Work out the finished part from the listing and answer in its coordinate system (mm). A direction names the side the tool comes from. Coordinates: 2 decimals unless noted, no trailing zeros. Order: outer loops, then holes, each group sorted by start corner. A loop starts at its lowest first (then second) coordinate and runs counter-clockwise, first axis right, second up. Notation, with made-up numbers: (-23.75, 61) - (0.25, 61) arc R23 ccw to (0.25, 72) - close; hole circle Ø5 at (74.25, 46). An arc over 180 degrees is marked (long way). Use CSV: the item, a comma, the result in double quotes. Start each with the question number.
from build123d import *

# Parameters (mm, degrees)
CYLINDER028_R          = 4
CYLINDER028_DEPTH      = 2.5
CYLINDER028_ROLL_ANGLE = 90
BOX023_W               = 5
BOX023_H               = 2.5
BOX023_DEPTH           = 2.5
CHAMFER003_SIZE        = 2.49
BOX021_W               = 5
BOX021_H               = 2.5
BOX021_DEPTH           = 2.5
CHAMFER001_SIZE        = 2.49
CYLINDER014_R          = 0.8
CYLINDER014_DEPTH      = 28
CYLINDER015_R          = 0.8
CYLINDER015_DEPTH      = 28
CYLINDER009_R          = 0.8
CYLINDER009_DEPTH      = 28
CYLINDER008_R          = 0.8
CYLINDER008_DEPTH      = 28
BOX012_W               = 73
BOX012_H               = 37
BOX012_DEPTH           = 3
BOX011_W               = 73
BOX011_H               = 3
BOX011_DEPTH           = 8
FILLET004_R            = 7.99
FILLET005_R            = 2


with BuildPart() as cylinder028:
    # Cylinder028 → Cylinder028 (new body)
    with BuildSketch(Plane.XY):
        Circle(CYLINDER028_R)
    extrude(amount=CYLINDER028_DEPTH)


with BuildPart() as cylinder028_1:
    # Cylinder028 roll: moved
    add(cylinder028.part.rotate(Axis((0, 0, 0), (1, 0, 0)), CYLINDER028_ROLL_ANGLE))


with BuildPart() as cylinder028_2:
    # Cylinder028 placement: moved
    add(cylinder028_1.part.moved(Location((63, 84.5, -17))))


with BuildPart() as chamfer003:
    # Box023 → Box023 (new body)
    with BuildSketch(Plane(origin=(70.5, 113, -22.5), x_dir=(1, 0, 0), z_dir=(0, 0, 1))):
        with Locations((2.5, 1.25)):
            Rectangle(BOX023_W, BOX023_H)
    extrude(amount=BOX023_DEPTH)

    # Chamfer003
    chamfer003_edges = [chamfer003.edges().sort_by_distance(p)[0] for p in [
        (73, 115.5, -22.5),
    ]]
    chamfer(chamfer003_edges, length=CHAMFER003_SIZE)


with BuildPart() as chamfer003_1:
    # Chamfer003 placement: moved
    add(chamfer003.part.moved(Location((55, 9, 0))))


with BuildPart() as fusion016:
    # Box021 → Box021 (new body)
    with BuildSketch(Plane(origin=(70.5, 113, -22.5), x_dir=(1, 0, 0), z_dir=(0, 0, 1))):
        with Locations((2.5, 1.25)):
            Rectangle(BOX021_W, BOX021_H)
    extrude(amount=BOX021_DEPTH)

    # Chamfer001
    chamfer001_edges = [fusion016.edges().sort_by_distance(p)[0] for p in [
        (73, 115.5, -22.5),
    ]]
    chamfer(chamfer001_edges, length=CHAMFER001_SIZE)


with BuildPart() as fusion016_1:
    # Chamfer001 placement: moved
    add(fusion016.part.moved(Location((1, 9, 0))))

    # Fusion016: union Chamfer003
    add(chamfer003_1.part)


with BuildPart() as cylinder014:
    # Cylinder014 → Cylinder014 (new body)
    with BuildSketch(Plane(origin=(74, 118, -26), x_dir=(1, 0, 0), z_dir=(0, 0, 1))):
        Circle(CYLINDER014_R)
    extrude(amount=CYLINDER014_DEPTH)


with BuildPart() as fusion011:
    # Cylinder015 → Cylinder015 (new body)
    with BuildSketch(Plane(origin=(74, 94, -26), x_dir=(1, 0, 0), z_dir=(0, 0, 1))):
        Circle(CYLINDER015_R)
    extrude(amount=CYLINDER015_DEPTH)

    # Fusion011: union Cylinder014
    add(cylinder014.part)


with BuildPart() as fusion011_1:
    # Fusion011 placement: moved
    add(fusion011.part.moved(Location((54, 0, 0))))


with BuildPart() as cylinder009:
    # Cylinder009 → Cylinder009 (new body)
    with BuildSketch(Plane(origin=(74, 118, -26), x_dir=(1, 0, 0), z_dir=(0, 0, 1))):
        Circle(CYLINDER009_R)
    extrude(amount=CYLINDER009_DEPTH)


with BuildPart() as fusion012:
    # Cylinder008 → Cylinder008 (new body)
    with BuildSketch(Plane(origin=(74, 94, -26), x_dir=(1, 0, 0), z_dir=(0, 0, 1))):
        Circle(CYLINDER008_R)
    extrude(amount=CYLINDER008_DEPTH)

    # Fusion010: union Cylinder009
    add(cylinder009.part)

    # Fusion012: union Fusion011
    add(fusion011_1.part)


with BuildPart() as box012:
    # Box012 → Box012 (new body)
    with BuildSketch(Plane(origin=(64, 85, -23), x_dir=(1, 0, 0), z_dir=(0, 0, 1))):
        with Locations((36.5, 18.5)):
            Rectangle(BOX012_W, BOX012_H)
    extrude(amount=BOX012_DEPTH)


with BuildPart() as cut026:
    # Box011 → Box011 (new body)
    with BuildSketch(Plane(origin=(64, 82, -23), x_dir=(1, 0, 0), z_dir=(0, 0, 1))):
        with Locations((36.5, 1.5)):
            Rectangle(BOX011_W, BOX011_H)
    extrude(amount=BOX011_DEPTH)

    # Fusion001: union Box012
    add(box012.part)

    # Fillet004
    fillet004_edges = [cut026.edges().sort_by_distance(p)[0] for p in [
        (100.5, 82, -23),
    ]]
    fillet(fillet004_edges, radius=FILLET004_R)

    # Fillet005
    fillet005_edges = [cut026.edges().sort_by_distance(p)[0] for p in [
        (100.5, 85, -20),
    ]]
    fillet(fillet005_edges, radius=FILLET005_R)

    # Cut013: cut Fusion012
    add(fusion012.part, mode=Mode.SUBTRACT)

    # Fusion017: union Fusion016
    add(fusion016_1.part)

    # Cut026: cut Cylinder028
    add(cylinder028_2.part, mode=Mode.SUBTRACT)


solid = cut026.part
1) The part is cut by section A-A on y = 118. Determine the outline of the cut face in (x, z).
2) The part is cut by section C-C on z = -21.5. Determine the outline of the cut face in (x, y).
3) For a pull along Z with two mould halves and no side action, classify faces 1 (the face through (76.5, 123, -21)), 2 (the face through (66.932, 83.545, -17.735)), 3 (the face through (100, 106, -20)) as +Z half, -Z half, draft (parallel to the pull), parting line (faces both ways), or undercut.
4) Flat-ended cylindrical pins translate along their axes: P1, Ø11, axis at x = 91, y = 97.5, coming from the +Z side; P2, Ø1.5, axis at x = 86.5, z = -17, coming from the +Y side; P3, Ø2, axis at x = 105, z = -17, coming from the -Y side; P4, Ø1, axis at x = 74, y = 94, coming from the -Z side. Find the tip coordinate at first contact, or state that the pin passes through.
5) Straight lines are drawn through the part: line 1 (X direction, y = 94, z = -21.2); line 2 (Y direction, x = 128, z = -20.75); line 3 (Z direction, x = 96.5, y = 98.5). For each, find the intervals that lie inside material, in ascending order. Write a range as [from, to].
6) The part is cut by section B-B on x = 128. State how many separate pieces and enclosed holes the cut face has, plus the area to 3 significant figures.
7) For faces 4 (the face through (65, 84.5, -17)), 5 (the face through (125.5, 123, -21)), 6 (the face through (130.5, 123, -21)), determine the directions among +Z, -Z, +X, -X, +Y, -Y from which every point of the face is accessible in a straight line to the end or side of a thin tool.
Answer key:
1,outline,"(64, -23) - (73.2, -23) - (73.2, -20) - (64, -20) - close; (74.8, -23) - (127.2, -23) - (127.2, -20) - (74.8, -20) - close; (128.8, -23) - (137, -23) - (137, -20) - (128.8, -20) - close"
2,outline,"(64, 85.33) - (137, 85.33) - (137, 122) - (130.5, 122) - (130.5, 123.01) - (125.5, 123.01) - (125.5, 122) - (76.5, 122) - (76.5, 123.01) - (71.5, 123.01) - (71.5, 122) - (64, 122) - close; hole circle Ø1.6 at (74, 94); hole circle Ø1.6 at (74, 118); hole circle Ø1.6 at (128, 94); hole circle Ø1.6 at (128, 118)"
3,face 1,"draft"
3,face 2,"undercut"
3,face 3,"+Z half"
4,P1,"z = -20"
4,P2,"y = 85"
4,P3,"y = 82.06"
4,P4,"through"
5,line 1,"[64, 73.2], [74.8, 127.2], [128.8, 137]"
5,line 2,"[84.43, 93.2], [94.8, 117.2], [118.8, 123.76]"
5,line 3,"[-23, -20]"
6,separate pieces,"3"
6,enclosed holes,"0"
6,area,"116 mm^2"
7,face 4,"-X, -Y"
7,face 5,"+Z, -Z, +Y"
7,face 6,"+Z, -Z, +X, +Y"
